Input: part model. Units: mm. Frame: model coordinates. Coordinates: 2 decimals unless noted, no trailing zeros. Write each loop counter-clockwise with the first axis right and the second up, starting at its lowest first coordinate (ties: lowest second). Pieces come first, ordered by that corner, then holes.
from build123d import *

# Parameters (mm, degrees)
F0_R     = 3
F1_DEPTH = 10
F2_W     = 114.1267567873
F2_H     = 80.1076181233
F3_DEPTH = 5


with BuildPart() as f1:
    # F0 (on Top) → F1 (new body)
    with BuildSketch(Plane.XY):
        with Locations((-49, 0)):
            Circle(F0_R)
    extrude(amount=F1_DEPTH)



with BuildPart() as f1b:
    # F0 (on Top) → F1, piece 2 (new body)
    with BuildSketch(Plane.XY):
        with BuildLine():
            ThreePointArc((-3, 0), (0, -3), (3, 0))
            ThreePointArc((3, 0), (0, 3), (-3, 0))
        make_face()
    extrude(amount=F1_DEPTH)


with BuildPart() as f1_1:
    add(f1.part)

    add(f1b.part)  # F3 merges F1b
    # F2 (on Top) → F3 (join)
    with BuildSketch(Plane.XY):
        with Locations((-1.3738982379, 1.3595465571)):
            Rectangle(F2_W, F2_H)
    extrude(amount=-F3_DEPTH)


solid = f1_1.part
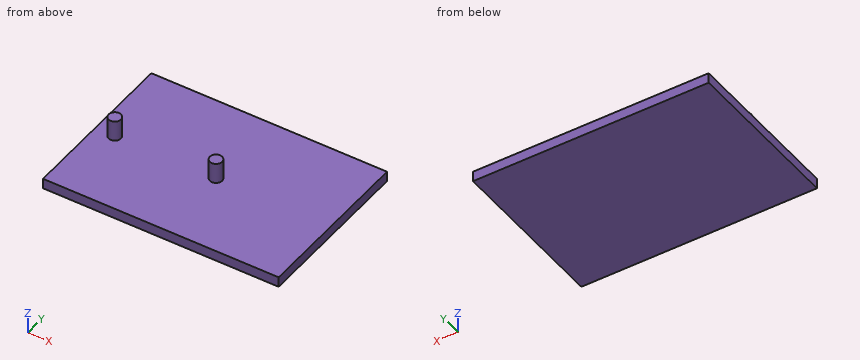
Item 1: Pin query (flat end, axial travel): pin 1 Ø2 at (x, y) = (20, 13.5) entering from +Z. Return the tip coordinate at first contact, or that it passes through.
Item 2: Material intervals for line 1 (Z direction, x = 48.5, y = 35); line 2 (X direction, y = 2, z = 9); line 3 (Y direction, x = -49, z = 4.75), sorted ascending.
Item 3: Section query A-A, the plane y = 0. Return loops of the section in (x, z).
Item 4: Section query B-B, the plane x = 0. Return loops of the section in (y, z), then the cut area to 3 significant figures.
Item 5: Section query D-D, the plane x = -49.5. Return loops of the section in (y, z), then the cut area to 3 significant figures.
Item 6: Section query C-C, the plane z = 8.25. Return loops of the section in (x, y).
The answers:
1. pin 1: stops at z = 0
2. line 1: z = -5 to 0
2. line 2: x = -51.24 to -46.76, -2.24 to 2.24
2. line 3: y = -3 to 3
3. outline: (-58.44, -5) - (55.69, -5) - (55.69, 0) - (3, 0) - (3, 10) - (-3, 10) - (-3, 0) - (-46, 0) - (-46, 10) - (-52, 10) - (-52, 0) - (-58.44, 0) - close
4. outline: (-38.69, -5) - (41.41, -5) - (41.41, 0) - (3, 0) - (3, 10) - (-3, 10) - (-3, 0) - (-38.69, 0) - close
4. area: 461 mm2
5. outline: (-38.69, -5) - (41.41, -5) - (41.41, 0) - (2.96, 0) - (2.96, 10) - (-2.96, 10) - (-2.96, 0) - (-38.69, 0) - close
5. area: 460 mm2
6. outline: circle Ø6 at (-49, 0); circle Ø6 at (0, 0)
